Part model, mm, in its own coordinate system. A direction names the side the tool comes from. Coordinates: 2 decimals unless noted, no trailing zeros. Write each loop counter-clockwise with the first axis right and the second up, starting at its lowest first coordinate (ties: lowest second). Pieces come first, ordered by that corner, then holes. Notation, with made-up numbers: M -37.5,19.25 L -29.5,19.25 A7 cw -29.5,27.25 Z; hole C 89,78.25 d7. An arc over 180 degrees is marked long. Use a Markdown table: item, result. Add a question column.
Q1. Pin check, flat tips, straight feed: pin 1 Ø12 at (x, z) = (-34.72, 12.7) entering from +Y; pin 2 Ø12 at (y, z) = (30.04, 12.7) entering from +X; pin 3 Ø10 at (x, y) = (-19, 50) entering from +Z; pin 4 Ø9 at (y, z) = (30.04, 12.7) entering from -X. Stop position of each tip, or through.
Q2. Slice it at C-C on x = -35. Write the cut outline in (y, z), then the cut area to 3 significant figures.
Q3. Tool access for faces 5 (the cylindrical face through (-39.411, 49.003, 3.686)), 6 (the cylindrical face through (-53.684, 22.774, 14.989)), 7 (the flat face through (-43.4, 35.9, 25.4)), 8 (the flat face through (-22.023, 24, 4)): list every direction of +Z, -Z, +X, -X, +Y, -Y with a clear straight run to the whole face (end or side of a thin tool).
Q4. Slice it at B-B on y = 46. Write the cut outline in (x, z).
Q5. Wall check: L1, parallel to X at y = 19.5, z = 8; L2, parallel to Y at x = -30, z = 17; L3, parallel to Z at x = -28.5, y = 41. Give the ranges that are in metal, low to high. Write a range as from..to.
Q6. Mould opens along Z. For faces 1 (the cylindrical face through (-27.11, 49, 13.04)), 2 (the flat face through (-47.423, 30, 13)), 3 (the flat face through (-35, 30, 0)), 4 (the flat face through (-33, 38, 38.1)) say: released by +Z, released by -Z, zero draft, split by the parting line, or undercut.
Q7. Slice it at D-D on x = -53.5. Write the cut outline in (y, z), then the cut area to 3 significant figures.
Q8. Slice it at A-A on z = 12.7. Write the cut outline in (x, y).
from build123d import *

# Parameters (mm, degrees)
F0_W     = 25.4
F0_H     = 25.4
F1_DEPTH = 25.4
F3_R     = 10.16
F3_R_2   = 7.62
F4_DEPTH = 12.7
F5_R     = 10.16
F5_R_2   = 7.62
F7_DEPTH = 12.7
F6_R     = 10.16
F6_R_2   = 7.62
F8_DEPTH = 12.7
F2_R     = 10.16
F2_R_2   = 7.62
F9_DEPTH = 12.7


with BuildPart() as f1:
    # F0 (on Top) → F1 (new body)
    with BuildSketch(Plane.XY):
        with Locations((-34.72263, 30.04187)):
            Rectangle(F0_W, F0_H)
    extrude(amount=F1_DEPTH)

    # F3 (on face) → F4 (join)
    with BuildSketch(Plane(origin=(0, 42.74187, 0), x_dir=(-1, 0, 0), z_dir=(0, 1, 0))):
        with Locations((34.72263, 12.7)):
            Circle(F3_R)
        with Locations((34.72263, 12.7)):
            Circle(F3_R_2, mode=Mode.SUBTRACT)
    extrude(amount=F4_DEPTH)

    # F5 (on face) → F7 (join)
    with BuildSketch(Plane.XY.offset(25.4)):
        with Locations((-34.72263, 30.04187)):
            Circle(F5_R)
        with Locations((-34.72263, 30.04187)):
            Circle(F5_R_2, mode=Mode.SUBTRACT)
    extrude(amount=F7_DEPTH)

    # F6 (on face) → F8 (join)
    with BuildSketch(Plane(origin=(-47.42263, 0, 0), x_dir=(0, -1, 0), z_dir=(-1, 0, 0))):
        with Locations((-30.04187, 12.7)):
            Circle(F6_R)
        with Locations((-30.04187, 12.7)):
            Circle(F6_R_2, mode=Mode.SUBTRACT)
    extrude(amount=F8_DEPTH)

    # F2 (on face) → F9 (join)
    with BuildSketch(Plane.YZ.offset(-22.02263)):
        with Locations((30.04187, 12.7)):
            Circle(F2_R)
        with Locations((30.04187, 12.7)):
            Circle(F2_R_2, mode=Mode.SUBTRACT)
    extrude(amount=F9_DEPTH)


solid = f1.part
Recorded:
| question | item | result |
|---|---|---|
| 1 | pin 1 | y = 42.74 |
| 1 | pin 2 | x = -22.02 |
| 1 | pin 3 | through |
| 1 | pin 4 | x = -47.42 |
| 2 | outline | M 17.34,0 L 42.74,0 L 42.74,2.54 L 55.44,2.54 L 55.44,5.09 L 42.74,5.09 L 42.74,20.31 L 55.44,20.31 L 55.44,22.86 L 42.74,22.86 L 42.74,25.4 L 40.2,25.4 L 40.2,38.1 L 37.66,38.1 L 37.66,25.4 L 22.43,25.4 L 22.43,38.1 L 19.89,38.1 L 19.89,25.4 L 17.34,25.4 Z |
| 2 | area | 774 mm² |
| 3 | face 5 | +Y |
| 3 | face 6 | -X |
| 3 | face 7 | +Z |
| 3 | face 8 | +X |
| 4 | outline | C -34.72,12.7 d20.32; hole C -34.72,12.7 d15.24 |
| 5 | L1 | -47.42..-22.02 |
| 5 | L2 | 17.34..42.74 |
| 5 | L3 | 0..25.4 |
| 6 | face 1 | undercut |
| 6 | face 2 | undercut |
| 6 | face 3 | released by -Z |
| 6 | face 4 | released by +Z |
| 7 | outline | C 30.04,12.7 d20.32; hole C 30.04,12.7 d15.24 |
| 7 | area | 142 mm² |
| 8 | outline | M -60.12,19.88 L -47.42,19.88 L -47.42,17.34 L -22.02,17.34 L -22.02,19.88 L -9.32,19.88 L -9.32,22.42 L -22.02,22.42 L -22.02,37.66 L -9.32,37.66 L -9.32,40.2 L -22.02,40.2 L -22.02,42.74 L -24.56,42.74 L -24.56,55.44 L -27.1,55.44 L -27.1,42.74 L -42.34,42.74 L -42.34,55.44 L -44.88,55.44 L -44.88,42.74 L -47.42,42.74 L -47.42,40.2 L -60.12,40.2 L -60.12,37.66 L -47.42,37.66 L -47.42,22.42 L -60.12,22.42 Z |
